The model under review builds one solid part; all positions refer to its coordinate system, in mm. Face numbers are marked on the shaded views. A direction names the side the tool comes from. Coordinates: 2 decimals unless noted, no trailing zeros. Order: outer loops, then holes, each group sorted by start corner. A loop starts at its lowest first (then second) coordinate and runs counter-clockwise, first axis right, second up. Notation, with made-up numbers: (62, -20.75) -> (90, -20.75) arc R31 cw to (90, 9.25) -> close; hole circle Ø7 at (8, 86). An arc over 180 degrees is marked (long way). Put each result on its own line as item: value.
from build123d import *

# Parameters (mm, degrees)
M12X1_5_TAPPED_HOLE1_D           = 10.5
M12X1_5_TAPPED_HOLE1_DEPTH       = 24.84548175
M12X1_5_TAPPED_HOLE1_CSINK_D     = 12.05
M12X1_5_TAPPED_HOLE1_CSINK_ANGLE = 90
M12X1_5_TAPPED_HOLE1_TIP         = 3.15451825


with BuildPart() as part:
    # Sketch1 → Revolve1 (revolve)
    with BuildSketch(Plane.XY, mode=Mode.PRIVATE) as revolve1_sk:
        Polygon((0, 11), (14, 11), (14, 22.5), (24, 32.5), (74, 32.5), (84, 22.5), (84, 19), (249, 19), (249, 0), (0, 0), align=None)
    revolve(revolve1_sk.sketch.rotate(Axis((0, 0, 0), (1, 0, 0)), 90), axis=Axis((0, 0, 0), (1, 0, 0)))

    # M12x1.5 Tapped Hole1
    with Locations(Plane(origin=(0, 0, 0), x_dir=(0, 0, -1), z_dir=(-1, 0, 0))):
        with Locations((0, 0)):
            CounterSinkHole(M12X1_5_TAPPED_HOLE1_D / 2, M12X1_5_TAPPED_HOLE1_CSINK_D / 2, depth=M12X1_5_TAPPED_HOLE1_DEPTH, counter_sink_angle=M12X1_5_TAPPED_HOLE1_CSINK_ANGLE)
            with Locations((0, 0, -(M12X1_5_TAPPED_HOLE1_DEPTH + M12X1_5_TAPPED_HOLE1_TIP / 2))):  # 118° drill point
                Cone(0, M12X1_5_TAPPED_HOLE1_D / 2, M12X1_5_TAPPED_HOLE1_TIP, mode=Mode.SUBTRACT)


solid = part.part
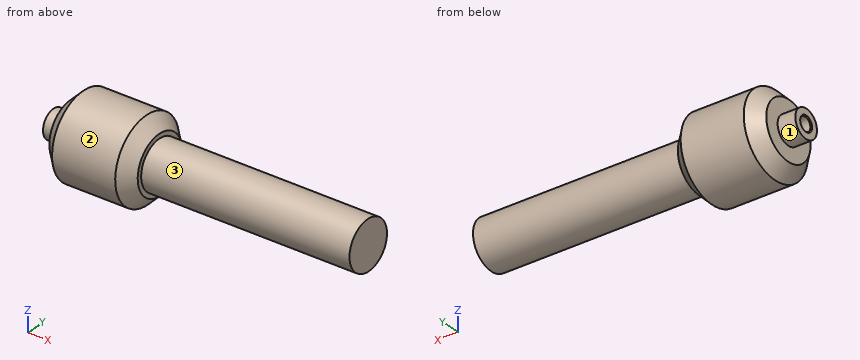
Item 1: Consider section A-A on x = 198.5. Write out the cut boundary in (y, z).
Answers below:
outline: circle Ø38 at (0, 0)
Item 2: For the marked faces 1, 2 and 3, list the 3-axis set-ups (+Z, -Z, +X, -X, +Y, -Y) from which the entire face can be reached by the end or side of a thin tool; tool diameter is ignored.
Answers below:
face 1: -X
face 2: +X, -X
face 3: +X
Item 3: For line 1 (Y direction, x = 7.25, z = 0); line 2 (X direction, y = -4, z = 15.5); line 3 (X direction, y = 2, z = -22), list the stretches that pass through material, from the lowest coordinate up. Write a range as from..to.
Answers below:
line 1: -11..-5.25, 5.25..11
line 2: 14..249
line 3: 14..84
Item 4: For pin 1 Ø13.5 at (y, z) = (-4.5, 7.5) entering from -X; pin 2 Ø6 at (x, y) = (128, 12.5) entering from +Z; pin 3 Ø2 at (x, z) = (214.5, -3) entering from -Y; pin 4 Ø3 at (x, y) = (44, 17.5) entering from +Z, all flat-tipped, find the tip position at first contact; note any pin that passes through.
Answers below:
pin 1: x = 0
pin 2: z = 16.45
pin 3: y = -18.89
pin 4: z = 28.29
Item 5: Consider section B-B on x = 40. Write out the cut boundary in (y, z).
Answers below:
outline: circle Ø65 at (0, 0)
